Check sheet for the drawn part. Datum: minimum x, y, z corner. Units: mm. Give positions to 0.01 mm unless a question says otherwise; leave off trailing zeros. Write each loop counter-clockwise with the first axis right and the second up, starting at its lowest first coordinate (ties: lowest second). Pieces come first, ordered by that corner, then holes. Notation, with made-up numbers: (57, -24) - (76, -24) arc R24 ccw to (76, 2) - close; hole circle Ø1 at (24.5, 82.25). An arc over 180 degrees is marked (long way). Return JSON: item names as keys, results as strings. Group by question number.
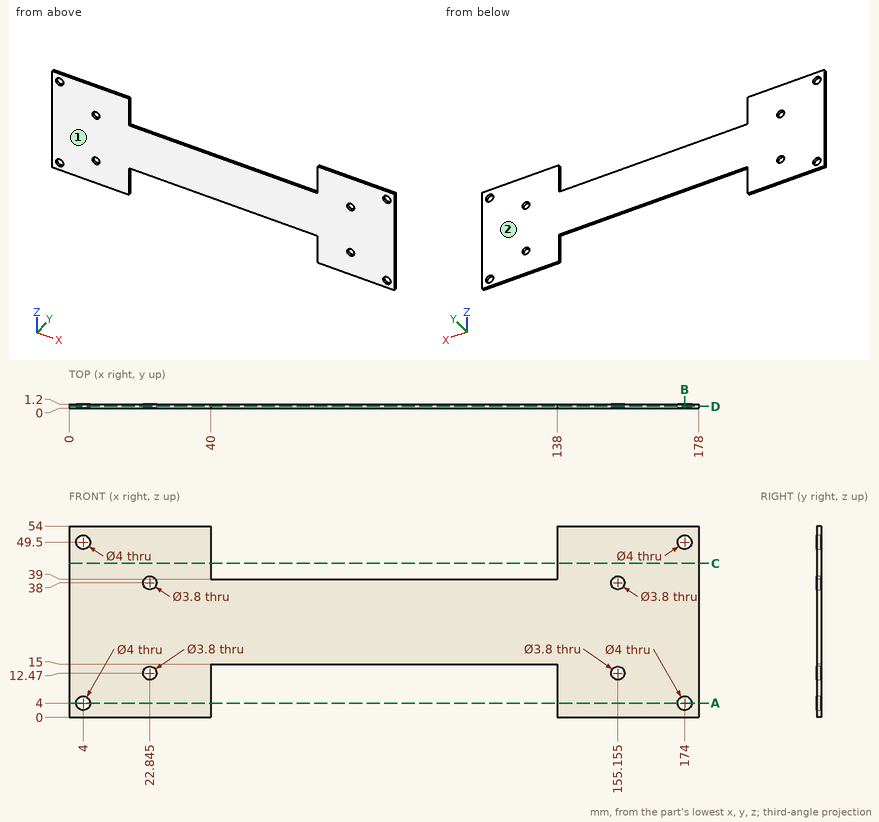
Item 1: Section check B-B on x = 174. Record the cut outline in (y, z), plus the area to 3 significant figures.
Item 2: Material ranges on line 1 along Z through (x, y) = (174, 0.65); line 2 along X through (y, z) = (0.6, 4); line 3 along X through (y, z) = (0.5, 38) (3 decimals), recorded low to high. Write a range as from..to.
Item 3: Section check D-D on y = 0.55. Count the separate pieces of the cut face and the enclosed holes in it, plus the area to 3 significant figures.
Item 4: Section check C-C on z = 43.5. Record the cut outline in (x, y), plus the area to 3 significant figures.
Item 5: Section check A-A on z = 4. Record the cut outline in (x, y), plus the area to 3 significant figures.
Item 6: Mould release check, pull along Y, two halves, no side actions. Record for the marked faces 1 and 2: +Y half, -Y half, draft (parallel to the pull), parting line (faces both ways), or undercut.
Reply:
{
 "1": {"outline": "(0, 0) - (1.2, 0) - (1.2, 2) - (0, 2) - close; (0, 6) - (1.2, 6) - (1.2, 47.5) - (0, 47.5) - close; (0, 51.5) - (1.2, 51.5) - (1.2, 54) - (0, 54) - close", "area": "55.2 mm²"},
 "2": {"line 1": "0..2, 6..47.5, 51.5..54", "line 2": "0..2, 6..40, 138..172, 176..178", "line 3": "0..20.945, 24.745..153.255, 157.055..178"},
 "3": {"separate pieces": "1", "enclosed holes": "8", "area": "6,580 mm²"},
 "4": {"outline": "(0, 0) - (40, 0) - (40, 1.2) - (0, 1.2) - close; (138, 0) - (178, 0) - (178, 1.2) - (138, 1.2) - close", "area": "96.0 mm²"},
 "5": {"outline": "(0, 0) - (2, 0) - (2, 1.2) - (0, 1.2) - close; (6, 0) - (40, 0) - (40, 1.2) - (6, 1.2) - close; (138, 0) - (172, 0) - (172, 1.2) - (138, 1.2) - close; (176, 0) - (178, 0) - (178, 1.2) - (176, 1.2) - close", "area": "86.4 mm²"},
 "6": {"face 1": "-Y half", "face 2": "+Y half"}
}
